The listing builds one solid part. Answer for the finished solid, in the listing's coordinates (mm). A direction names the side the tool comes from. Coordinates: 2 decimals unless noted, no trailing zeros. Write each loop counter-clockwise with the first axis right and the second up, starting at its lowest first coordinate (ties: lowest second). Pieces come first, ordered by that corner, then holes.
from build123d import *

# Parameters (mm, degrees)
SKETCH_R        = 11
PAD_DEPTH       = 12.5
SKETCH001_R     = 2.75
POCKET_DEPTH    = 25.001
SKETCH002_R     = 5
POCKET001_DEPTH = 7
SKETCH003_R     = 2.75
POCKET002_DEPTH = 39.001
CHAMFER_SIZE    = 1
CHAMFER005_SIZE = 0.5
CHAMFER006_SIZE = 0.5
CHAMFER007_SIZE = 0.5
CHAMFER008_SIZE = 0.5
CHAMFER009_SIZE = 0.5
SKETCH004_W     = 33
SKETCH004_H     = 33
SKETCH004_R     = 11
PAD001_DEPTH    = 6.5
CHAMFER003_SIZE = 1
CHAMFER004_SIZE = 0.5


with BuildPart() as bearing:
    # Sketch005 → Revolution (revolve)
    with BuildSketch(Plane.YZ):
        Polygon((-20, 27), (13.5, 27), (13.5, 29), (12.5, 29), (12.5, 33), (-19, 33), (-19, 29), (-20, 29), align=None)
    revolve(axis=Axis((0, -30, 22), (0, 1, 0)))


with BuildPart() as housing_bearing_hole_chamfer:
    # Sketch → Pad (new body, symmetric)
    with BuildSketch(Plane.XZ):
        Polygon((-30, 0), (-30, 32.5), (-17, 32.5), (-17, 39), (17, 39), (17, 32.5), (30, 32.5), (30, 0), align=None)
        with Locations((0, 22)):
            Circle(SKETCH_R, mode=Mode.SUBTRACT)
    extrude(amount=PAD_DEPTH, both=True)

    # Sketch001 → Pocket (cut, through all)
    with BuildSketch(Plane.XZ.offset(12.5)):
        with Locations((-23, 22)):
            Circle(SKETCH001_R)
        with Locations((23, 22)):
            Circle(SKETCH001_R)
        with Locations((-23, 7)):
            Circle(SKETCH001_R)
        with Locations((23, 7)):
            Circle(SKETCH001_R)
    extrude(amount=-POCKET_DEPTH, mode=Mode.SUBTRACT)

    # Sketch002 → Pocket001 (cut)
    with BuildSketch(Plane(origin=(0, 0, 32.5), x_dir=(-1, 0, 0), z_dir=(0, 0, 1))):
        with Locations((-23, 6.5)):
            Circle(SKETCH002_R)
        with Locations((23, 6.5)):
            Circle(SKETCH002_R)
        with Locations((-23, -6.5)):
            Circle(SKETCH002_R)
        with Locations((23, -6.5)):
            Circle(SKETCH002_R)
    extrude(amount=-POCKET001_DEPTH, mode=Mode.SUBTRACT)

    # Sketch003 → Pocket002 (cut, through all)
    with BuildSketch(Plane(origin=(0, 0, 0), x_dir=(1, 0, 0), z_dir=(0, 0, -1))):
        with Locations((-23, 6.5)):
            Circle(SKETCH003_R)
        with Locations((23, 6.5)):
            Circle(SKETCH003_R)
        with Locations((-23, -6.5)):
            Circle(SKETCH003_R)
        with Locations((23, -6.5)):
            Circle(SKETCH003_R)
    extrude(amount=-POCKET002_DEPTH, mode=Mode.SUBTRACT)

    # Chamfer
    chamfer_edges = [housing_bearing_hole_chamfer.edges().sort_by_distance(p)[0] for p in [
        (17, 0, 39),
        (0, 12.5, 39),
        (-17, 0, 39),
        (0, -12.5, 39),
    ]]
    chamfer(chamfer_edges, length=CHAMFER_SIZE)

    # Chamfer005
    chamfer005_edges = [housing_bearing_hole_chamfer.edges().sort_by_distance(p)[0] for p in [
        (30, -12.5, 16.25),
        (30, 0, 32.5),
        (30, 12.5, 16.25),
        (30, 0, 0),
        (0, -12.5, 0),
        (0, 12.5, 0),
        (-30, 0, 0),
        (-30, -12.5, 16.25),
        (-30, 12.5, 16.25),
        (-30, 0, 32.5),
    ]]
    chamfer(chamfer005_edges, length=CHAMFER005_SIZE)

    # Chamfer006
    chamfer006_edges = [housing_bearing_hole_chamfer.edges().sort_by_distance(p)[0] for p in [
        (-18, -6.5, 32.5),
        (-18, 6.5, 32.5),
        (28, 6.5, 32.5),
        (28, -6.5, 32.5),
    ]]
    chamfer(chamfer006_edges, length=CHAMFER006_SIZE)

    # Chamfer007
    chamfer007_edges = [housing_bearing_hole_chamfer.edges().sort_by_distance(p)[0] for p in [
        (-25.75, -6.5, 0),
        (20.25, -6.5, 0),
        (20.25, 6.5, 0),
        (-25.75, 6.5, 0),
    ]]
    chamfer(chamfer007_edges, length=CHAMFER007_SIZE)

    # Chamfer008
    chamfer008_edges = [housing_bearing_hole_chamfer.edges().sort_by_distance(p)[0] for p in [
        (20.25, -12.5, 22),
        (-25.75, -12.5, 22),
        (-25.75, -12.5, 7),
        (20.25, -12.5, 7),
        (20.25, 12.5, 22),
        (20.25, 12.5, 7),
        (-25.75, 12.5, 22),
        (-25.75, 12.5, 7),
    ]]
    chamfer(chamfer008_edges, length=CHAMFER008_SIZE)

    # Chamfer009
    chamfer009_edges = [housing_bearing_hole_chamfer.edges().sort_by_distance(p)[0] for p in [
        (-11, 12.5, 22),
    ]]
    chamfer(chamfer009_edges, length=CHAMFER009_SIZE)


with BuildPart() as bk10:
    # Sketch004 → Pad001 (new body)
    with BuildSketch(Plane.XZ.offset(12.5)):
        with Locations((0, 22)):
            Rectangle(SKETCH004_W, SKETCH004_H)
        with Locations((0, 22)):
            Circle(SKETCH004_R, mode=Mode.SUBTRACT)
    extrude(amount=PAD001_DEPTH)

    # Chamfer003
    chamfer003_edges = [bk10.edges().sort_by_distance(p)[0] for p in [
        (16.5, -15.75, 38.5),
        (-16.5, -15.75, 38.5),
        (-16.5, -15.75, 5.5),
        (16.5, -15.75, 5.5),
    ]]
    chamfer(chamfer003_edges, length=CHAMFER003_SIZE)

    # Chamfer004
    chamfer004_edges = [bk10.edges().sort_by_distance(p)[0] for p in [
        (-11, -19, 22),
    ]]
    chamfer(chamfer004_edges, length=CHAMFER004_SIZE)

    # Fusion: union housing-bearing-hole-chamfer
    add(housing_bearing_hole_chamfer.part)

    # Fusion001: union bearing
    add(bearing.part)


solid = bk10.part
1. Flat-ended cylindrical pins translate along their axes: P1, Ø9, axis at x = 23, z = 22, coming from the +Y side; P2, Ø3, axis at x = -23.5, y = -9, coming from the +Z side; P3, Ø11, axis at x = -23.5, y = 7, coming from the +Z side. Find the tip coordinate at first contact, or state that the pin passes through.
Results found:
P1: stops at y = 12.5
P2: stops at z = 25.5
P3: stops at z = 32.5
2. Section A-A on z = 35.5 is taken. Give the vertices of the cut face in (x, y).
Results found:
outline: (-17, -12.5) - (-16.5, -12.5) - (-16.5, -19) - (16.5, -19) - (16.5, -12.5) - (17, -12.5) - (17, 12.5) - (-17, 12.5) - close
3. Find the intervals of material crossed by L1, parallel to Y at x = -23, z = 27.25; L2, parallel to Z at x = 23, y = -9.9; L3, parallel to Y at x = 23, z = 2.75, in increasing order.
Results found:
L1: y = -12.5 to -11.5, -1.5 to 1.5, 11.5 to 12.5
L2: z = 0 to 4.25, 9.75 to 19.25, 24.75 to 25.5
L3: y = -12.5 to -9.25, -3.75 to 3.75, 9.25 to 12.5
4. Section B-B on x = 23 is taken. State how many separate pieces and enclosed holes the cut face has, then the cut area to 3 significant figures.
Results found:
separate pieces: 9
enclosed holes: 0
area: 236 mm2
5. A tool of negligible diameter and unlimited length cuts with its end or side. For faces 1 (the flat face through (21, -4, 25.5)), 2 (the cylindrical face through (0, 13, 15)), 3 (the flat face through (0, -12.5, 3)), 4 (the flat face through (0.2, -19, 29.2)), from which of +Z, -Z, +X, -X, +Y, -Y can it reach the whole face along a straight path? Write none if from no direction.
Results found:
face 1: +Z
face 2: +Y
face 3: -Z, -Y
face 4: -Y
6. For a pull along X with two mould halves and no side action, classify faces 5 (the flat face through (16.5, -16, 22)), 6 (the flat face through (0.2, 12.5, 14.8)), 7 (the cylindrical face through (20.253, -6.621, 24.503)) as pulls with the +X half, pulls with the -X half, needs draft (parallel to the pull), parting line crosses it, or undercut.
Results found:
face 5: pulls with the +X half
face 6: needs draft
face 7: undercut
